from build123d import *

# Parameters (mm, degrees)
BOSS_EXTRUDE1_DEPTH = 7.62
SKETCH4_W           = 6.35
SKETCH4_H           = 34.925
BOSS_EXTRUDE3_DEPTH = 12.7
SKETCH5_R           = 11.1125
CUT_EXTRUDE1_DEPTH  = 12.7
SKETCH6_W           = 25.4
SKETCH6_H           = 3.175
BOSS_EXTRUDE4_DEPTH = 3.175
SKETCH7_W           = 25.4
SKETCH7_H           = 3.175
BOSS_EXTRUDE5_DEPTH = 3.175
SKETCH10_W          = 6.35
SKETCH10_H          = 34.925
BOSS_EXTRUDE8_DEPTH = 9.525
FILLET1_R           = 2
FILLET2_R           = 2
SKETCH11_R          = 17.4625
BOSS_EXTRUDE9_DEPTH = 19.05
SKETCH12_R          = 11.1125
CUT_EXTRUDE2_DEPTH  = 47.677899348
FILLET3_R           = 1
FILLET4_R           = 3


with BuildPart() as part:
    # Sketch1 → Boss-Extrude1 (new body)
    with BuildSketch(Plane(origin=(0, 0, 0), x_dir=(1, 0, 0), z_dir=(0, 1, 0))):
        with BuildLine():
            Line((37.1475, -17.4625), (37.1475, 17.4625))
            Line((37.1475, 17.4625), (-19.685, 17.4625))
            ThreePointArc((-19.685, 17.4625), (-37.1475, 0), (-19.685, -17.4625))
            Line((-19.685, -17.4625), (37.1475, -17.4625))
        make_face()
    extrude(amount=BOSS_EXTRUDE1_DEPTH)

    # Sketch4 → Boss-Extrude3 (add)
    with BuildSketch(Plane(origin=(0, 7.62, 0), x_dir=(1, 0, 0), z_dir=(0, 1, 0))):
        with Locations((33.9725, 0)):
            Rectangle(SKETCH4_W, SKETCH4_H)
    extrude(amount=BOSS_EXTRUDE3_DEPTH)

    # Sketch5 → Cut-Extrude1 (cut)
    with BuildSketch(Plane(origin=(0, 7.62, 0), x_dir=(1, 0, 0), z_dir=(0, 1, 0))):
        with Locations(Location((-19.685, 0, 0), (0, 0, 270))):
            Circle(SKETCH5_R)
    extrude(amount=-CUT_EXTRUDE1_DEPTH, mode=Mode.SUBTRACT)

    # Sketch6 → Boss-Extrude4 (add)
    with BuildSketch(Plane(origin=(0, 7.62, 0), x_dir=(1, 0, 0), z_dir=(0, 1, 0))):
        with Locations((14.9225, 9.525)):
            Rectangle(SKETCH6_W, SKETCH6_H)
    extrude(amount=BOSS_EXTRUDE4_DEPTH)

    # Sketch7 → Boss-Extrude5 (add)
    with BuildSketch(Plane(origin=(0, 7.62, 0), x_dir=(1, 0, 0), z_dir=(0, 1, 0))):
        with Locations((14.9225, -9.525)):
            Rectangle(SKETCH7_W, SKETCH7_H)
    extrude(amount=BOSS_EXTRUDE5_DEPTH)

    # Sketch10 → Boss-Extrude8 (add)
    with BuildSketch(Plane(origin=(0, 20.32, 0), x_dir=(1, 0, 0), z_dir=(0, 1, 0))):
        with Locations((33.9725, 0)):
            Rectangle(SKETCH10_W, SKETCH10_H)
    extrude(amount=BOSS_EXTRUDE8_DEPTH)

    # Fillet1
    fillet1_edges = [part.edges().sort_by_distance(p)[0] for p in [
        (37.1475, 29.845, 0),
        (37.1475, 14.9225, -17.4625),
        (37.1475, 14.9225, 17.4625),
    ]]
    fillet(fillet1_edges, radius=FILLET1_R)

    # Fillet2
    fillet2_edges = [part.edges().sort_by_distance(p)[0] for p in [
        (-37.1475, 0, 0),
        (7.73125, 0, 17.4625),
        (37.1475, 0, 0),
        (7.73125, 0, -17.4625),
        (36.561713562, 0, -16.876713562),
        (36.561713562, 0, 16.876713562),
    ]]
    fillet(fillet2_edges, radius=FILLET2_R)

    # Sketch11 → Boss-Extrude9 (add)
    with BuildSketch(Plane(origin=(0, 7.62, 0), x_dir=(1, 0, 0), z_dir=(0, 1, 0))):
        with Locations(Location((-19.685, 0, 0), (0, 0, 270))):
            Circle(SKETCH11_R)
    extrude(amount=BOSS_EXTRUDE9_DEPTH)

    # Sketch12 → Cut-Extrude2 (cut, through all)
    with BuildSketch(Plane(origin=(0, 7.62, 0), x_dir=(-1, 0, 0), z_dir=(0, -1, 0))):
        with Locations(Location((19.685, 0, 0), (0, 0, 270))):
            Circle(SKETCH12_R)
    extrude(amount=-CUT_EXTRUDE2_DEPTH, mode=Mode.SUBTRACT)

    # Fillet3
    fillet3_edges = [part.edges().sort_by_distance(p)[0] for p in [
        (-19.685, 26.67, -11.1125),
        (-19.685, 0, -11.1125),
    ]]
    fillet(fillet3_edges, radius=FILLET3_R)

    # Fillet4
    fillet4_edges = [part.edges().sort_by_distance(p)[0] for p in [
        (-19.685, 26.67, -17.4625),
    ]]
    fillet(fillet4_edges, radius=FILLET4_R)


solid = part.part
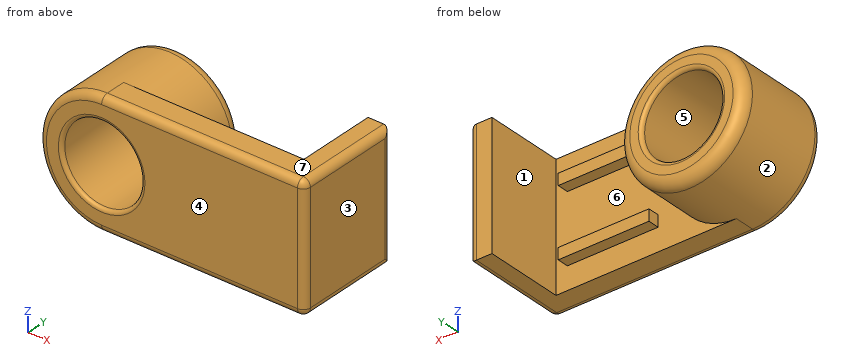
Geometry: final body of the model. Coordinates: model frame, mm. Face numbers are marked on the shaded views. A direction names the side the tool comes from. Give positions to 0.01 mm unless a question says otherwise; leave off trailing zeros. Order: outer loops, then holes, each group sorted by start corner. A loop starts at its lowest first (then second) coordinate and runs counter-clockwise, first axis right, second up. Notation, with made-up numbers: (14.5, 24) -> (19.5, 24) arc R18 cw to (19.5, 31) -> close; hole circle Ø9 at (-32.75, 20). An arc over 180 degrees is marked (long way). Put each result on its own line as item: value.
Q1. Section A-A, the plane y = 11.5. Return loops of the section in (x, z) (1 decimal), then the cut area to 3 significant figures.
Here are the results:
outline: circle Ø34.9 at (-19.7, 0); (30.8, -17.5) -> (35.1, -17.5) arc R2 ccw to (37.1, -15.5) -> (37.1, 15.5) arc R2 ccw to (35.1, 17.5) -> (30.8, 17.5) -> close; hole circle Ø22.2 at (-19.7, 0)
area: 790 mm^2
Q2. Reachability of the marked faces 1, 2 and 3 from +Z, -Z, +X, -X, +Y, -Y: full face, straight path, thin tool, end or side. Return the list, or none.
Here are the results:
face 1: +Z, -Z, +Y
face 2: +Y
face 3: +Z, -Z, +X, +Y, -Y
Q3. Material intervals for L1, parallel to X at y = 16.5, z = 0; L2, parallel to X at y = 19, z = 8; L3, parallel to Y at x = 17.5, z = -10 (3 decimals), sorted ascending.
Here are the results:
L1: x = -37.15 to -30.8, -8.57 to -2.22, 30.8 to 37.15
L2: x = -35.21 to -27.4, -11.97 to -4.16, 30.8 to 37.15
L3: y = 0 to 10.795
Q4. Section B-B, the plane y = 3.5. Return loops of the section in (x, z) (1 decimal), then the cut area to 3 significant figures.
Here are the results:
outline: (-19.7, -17.5) -> (35.1, -17.5) arc R2 ccw to (37.1, -15.5) -> (37.1, 15.5) arc R2 ccw to (35.1, 17.5) -> (-19.7, 17.5) arc R17.5 ccw to start; hole circle Ø22.2 at (-19.7, 0)
area: 2,070 mm^2
Q5. Section D-D, the plane x = 7. Return loops of the section in (y, z) (1 decimal).
Here are the results:
outline: (0, -15.5) arc R2 ccw to (2, -17.5) -> (7.6, -17.5) -> (7.6, -11.1) -> (10.8, -11.1) -> (10.8, -7.9) -> (7.6, -7.9) -> (7.6, 7.9) -> (10.8, 7.9) -> (10.8, 11.1) -> (7.6, 11.1) -> (7.6, 17.5) -> (2, 17.5) arc R2 ccw to (0, 15.5) -> close
Q6. Draft query along Z for the marked faces 4, 5, 6 and 7. Return one class per face: released by +Z, released by -Z, zero draft, split by the parting line, or undercut.
Here are the results:
face 4: zero draft
face 5: undercut
face 6: undercut
face 7: released by +Z
Q7. Pin query (flat end, axial travel): pin 1 (1.6 mm diameter, centred on x = 12.5, z = 10, fed in from +Y) (3 decimals); pin 2 (2 mm diameter, centred on y = 25.5, z = -4.5, fed in from -X); pin 3 (1.6 mm diameter, centred on y = 9.5, z = -9.5, fed in from -X). Return the tip coordinate at first contact, or that it passes through.
Here are the results:
pin 1: stops at y = 10.795
pin 2: stops at x = -36.52
pin 3: stops at x = -34.83
